Study the drawing (mm; zero at the part's minimum x, y, z) and answer. Coordinates: 2 decimals unless noted, no trailing zeros. Order: outer loops, then holes, each group sorted by start corner. A loop starts at its lowest first (then second) coordinate and runs counter-clockwise, first axis right, second up. Notation, with made-up numbers: (-37.75, 4) -> (-15.75, 4) arc R31 ccw to (-15.75, 38) -> close; hole circle Ø2 at (77.25, 40.5). An arc over 180 degrees is marked (long way). One line per question, with ' | ' between items.
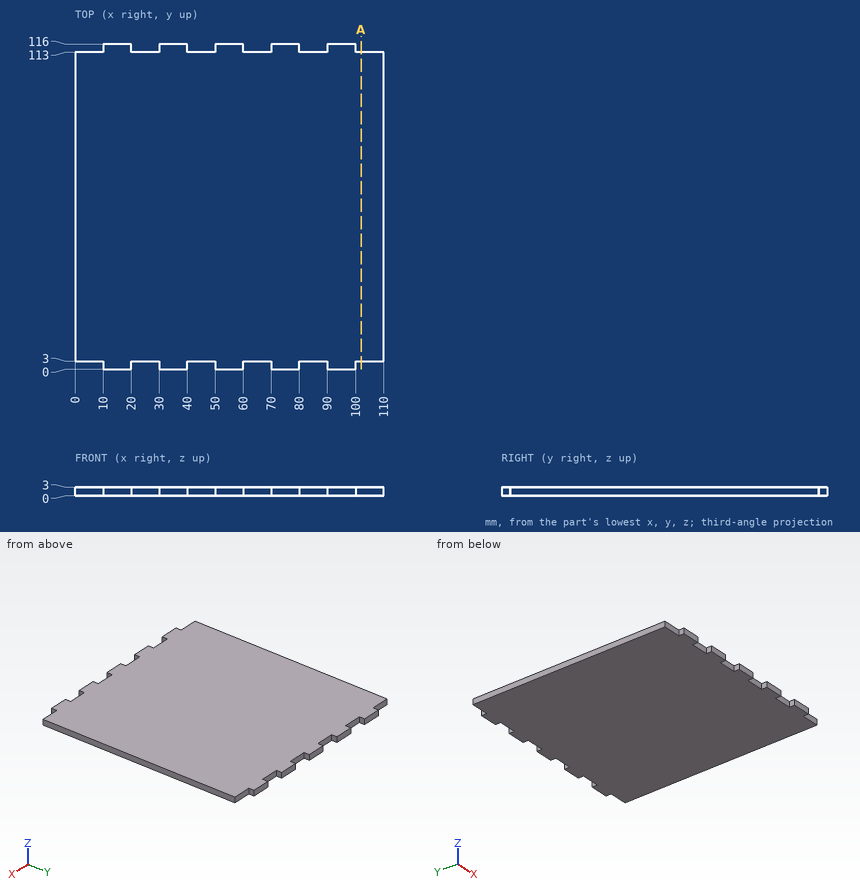
Item 1: Find the intervals of material crossed by L1, parallel to Y at x = 88.5, z = 2.05, in increasing order.
Computed values:
L1: y = 3 to 113
Item 2: Each of these flat-tipped pins is pushed along its axis until it touches: pin 1 Ø1.5 at (y, z) = (1, 1.5) entering from +X; pin 2 Ø1.5 at (x, z) = (87, 2) entering from -Y; pin 3 Ø0.9 at (y, z) = (1.5, 1.5) entering from -X; pin 4 Ø6 at (x, y) = (61, 54.5) entering from -Z. Where does it stop, or does it pass through?
Computed values:
pin 1: stops at x = 100 | pin 2: stops at y = 3 | pin 3: stops at x = 10 | pin 4: stops at z = 0
Item 3: Section A-A, the plane x = 102 is taken. Give the vertices of the cut face in (y, z), plus the area to 3 significant figures.
Computed values:
outline: (3, 0) -> (113, 0) -> (113, 3) -> (3, 3) -> close | area: 330 mm^2
